Can you work these out from the model? Positions are in its coordinate system, mm. A direction names the side the tool comes from. Coordinates: 2 decimals unless noted, no trailing zeros. Order: outer loops, then holes, each group sorted by start corner. A loop starts at its lowest first (then second) coordinate and runs counter-clockwise, first axis right, second up. Notation, with made-up numbers: (-36, 60.25) -> (-17, 60.25) arc R9 ccw to (-17, 65.25) -> close; hole circle Ø10 at (33, -29.5). An arc over 180 degrees is marked (long way). Use a Markdown table: item, result. Add a question column.
1. If I drill on line 1 along Z through (x, y) = (-35.5, 1.75); line 2 along Z through (x, y) = (-36.5, -1.75); line 3 along Z through (x, y) = (58, 7), over which ranges is the centre line in solid material (lowest first)? Write a range as from..to.
2. For pin 1 Ø5 at (y, z) = (-6.5, -9.5) entering from -X; pin 2 Ø10 at (x, y) = (-1.5, 2.5) entering from +Z; pin 3 Ø2 at (x, y) = (-17, 10) entering from -Z, each with a flat end and sliding along its axis, tell me the tip position at first contact or that it passes through.
3. Suppose I cut it at C-C, the plane y = -4. List the corners of the cut face in (x, z) for me.
4. Suppose I cut it at D-D, the plane x = -48.5. List the corners of the cut face in (y, z) for me, then the cut area to 3 significant figures.
5. Suppose I cut it at B-B, the plane x = -31. List the corners of the cut face in (y, z) for me.
6. We'd pull the mould along X, two halves only. Please class faces 1 (the flat face through (11, -12.5, 23)), 2 (the cylindrical face through (0.66, -0.175, -14.985)), 3 (the flat face through (-66.98, 0.18, -3.99)): pulls with the +X half, pulls with the -X half, needs draft (parallel to the pull), parting line crosses it, or undercut.
7. For faces 4 (the flat face through (-3.919, 0.175, 64.763)), 5 (the flat face through (11, 12.5, 23)), which set-ups out of +Z, -Z, +X, -X, +Y, -Y let a thin tool reach every point of the face, with its end or its side?
8. Suppose I cut it at A-A, the plane z = 0. List the corners of the cut face in (x, y) for me, then the cut area to 3 significant figures.
```python
from build123d import *

# Parameters (mm, degrees)
SKETCH_1_R      = 15
EXTRUDE_1_DEPTH = 12.5
FILLET_1_R      = 5


with BuildPart() as part:
    # 草图1 → 凸台-拉伸1 (new, symmetric)
    with BuildSketch(Plane(origin=(0, 0, 0), x_dir=(1, 0, 0), z_dir=(0, 1, 0))):
        with BuildLine():
            Line((-6.096427139, -65.918001187), (-1.679569826, -63.574633635))
            ThreePointArc((-1.679569826, -63.574633635), (0.953470582, -58.672633233), (-2.576772207, -54.371482736))
            Line((-2.576772207, -54.371482736), (-14.063876814, -50.900686325))
            Line((-14.063876814, -50.900686325), (-23.098048547, -33.872778153))
            ThreePointArc((-23.098048547, -33.872778153), (-32.102531801, -21.461490279), (-44.183478984, -12.018424012))
            Line((-44.183478984, -12.018424012), (-68.211524227, 1.854174377))
            Line((-68.211524227, 1.854174377), (-65.711524227, 6.184301396))
            ThreePointArc((-65.711524227, 6.184301396), (-28.145825623, 16.25), (-38.211524227, 53.815698604))
            Line((-38.211524227, 53.815698604), (-31.672954916, 65.14083286))
            ThreePointArc((-31.672954916, 65.14083286), (17.174057589, 15.576162499), (82.442373664, -8.563723486))
            ThreePointArc((82.442373664, -8.563723486), (88.420562961, -14.448425798), (84.460192724, -21.843284562))
            ThreePointArc((84.460192724, -21.843284562), (58.872866338, -40.770350543), (42.68980144, -68.175706017))
            ThreePointArc((42.68980144, -68.175706017), (20.995404286, -84.925315775), (-3.01984927, -71.716837758))
            Line((-3.01984927, -71.716837758), (-6.096427139, -65.918001187))
        make_face()
        with Locations(Location((0, 0, 0), (0, 0, 270))):
            Circle(SKETCH_1_R, mode=Mode.SUBTRACT)
    extrude(amount=EXTRUDE_1_DEPTH, both=True)

    # 圆角1
    fillet_1_edges = [part.edges().sort_by_distance(p)[0] for p in [
        (-31.672954916, 0, -65.14083286),
    ]]
    fillet(fillet_1_edges, radius=FILLET_1_R)


solid = part.part
```
Worked out:
| question | item | result |
|---|---|---|
| 1 | line 1 | z = -58.48..-52.03, -7.97..18.23 |
| 1 | line 2 | z = -56.78..-52.74, -7.26..17.38 |
| 1 | line 3 | z = 3.27..41.75 |
| 2 | pin 1 | stops at x = -36.89 |
| 2 | pin 2 | stops at z = 79.56 |
| 2 | pin 3 | stops at z = -46.44 |
| 3 | outline | (-68.21, -1.85) -> (-65.71, -6.18) arc R27.5 cw to (-38.21, -53.82) -> (-35.72, -58.14) arc R5 ccw to (-27.28, -58.5) arc R160 cw to (82.44, 8.56) arc R7 ccw to (84.46, 21.84) arc R80 cw to (42.69, 68.18) arc R25 ccw to (-3.02, 71.72) -> (-6.1, 65.92) -> (-1.68, 63.57) arc R5 cw to (-2.58, 54.37) -> (-14.06, 50.9) -> (-23.1, 33.87) arc R55 cw to (-44.18, 12.02) -> close; hole circle Ø30 at (0, 0) |
| 4 | outline | (-12.5, -2.72) -> (12.5, -2.72) -> (12.5, 9.53) -> (-12.5, 9.53) -> close |
| 4 | area | 306 mm² |
| 5 | outline | (-12.5, -60.62) -> (12.5, -60.62) -> (12.5, -47.8) -> (-12.5, -47.8) -> close; (-12.5, -12.2) -> (12.5, -12.2) -> (12.5, 22.64) -> (-12.5, 22.64) -> close |
| 6 | face 1 | needs draft |
| 6 | face 2 | undercut |
| 6 | face 3 | pulls with the -X half |
| 7 | face 4 | -X, +Y, -Y |
| 7 | face 5 | +Z, -Z, +X, -X, +Y |
| 8 | outline | (-65, -12.5) -> (-15, -12.5) -> (-15, 12.5) -> (-65, 12.5) -> close; (15, -12.5) -> (48.25, -12.5) -> (48.25, 12.5) -> (15, 12.5) -> close |
| 8 | area | 2,080 mm² |
